Geometry: final body of the model. Coordinates: model frame, mm. A direction names the side the tool comes from. Give positions to 0.01 mm unless a question says otherwise; leave off trailing zeros. Order: outer loops, then holes, each group sorted by start corner. A loop starts at its lowest first (then second) coordinate and runs counter-clockwise, first axis right, second up. Notation, with made-up numbers: (-18, 72.5) - (3, 72.5) arc R16 ccw to (3, 82.5) - close; hole circle Ø11 at (-4.75, 46). An arc over 180 degrees is marked (long way). Put each result on its own line as item: value. Start each with the question number.
1. Ray query, line 1 along Z through (x, y) = (12.5, -39); line 2 along Z through (x, y) = (23.5, -23); line 3 along Z through (x, y) = (12.5, -76). Return the intervals inside material, ascending. Write a range as from..to.
2. Mould query, pull axis Z, two halves, no side actions, for faces 1 (the flat face through (-0.07, -31.3, 76.04)), 2 (the flat face through (2, -38, 63.522)), 3 (the flat face through (-31, -38, -7.958)). Classes: pulls with the +Z half, pulls with the -Z half, needs draft (parallel to the pull), parting line crosses it, or undercut.
3. Section B-B on z = 35. Return the cut outline in (x, y), plus the area to 3 significant figures.
4. Section D-D on z = 58.5. Return the cut outline in (x, y).
5. Section A-A on z = -17. Return the cut outline in (x, y).
6. First-contact query: P1, Ø19, axis at y = -29, z = 30.5, coming from the -X side; P2, Ø12, axis at x = 20.5, y = -21, coming from the -Z side; P3, Ø8, axis at x = 22, y = -58.5, coming from the +Z side. Flat tips, straight axial feed; report the tip coordinate or a pass-through.
7. Section C-C on z = 13.5. Return the cut outline in (x, y).
8. Set-up query: faces 4 (the flat face through (-24.5, -39.2, 88.922)), 5 (the flat face through (-26.357, -49.706, 76.044)), 6 (the flat face through (-3.93, -24.06, 76.04)), 7 (the cylindrical face through (19.688, -13.873, 31.422)). Return all of +Z, -Z, +X, -X, +Y, -Y with unobstructed straight access to the full face (end or side cutting, diameter ignored); none if empty.
from build123d import *

# Parameters (mm, degrees)
F1_DEPTH  = 76.2
F2_R      = 25.4
F3_DEPTH  = 25.4
F5_DEPTH  = 25.4
F6_R      = 10.087603
F7_DEPTH  = 25.4
F9_DEPTH  = 25.4
F10_R     = 8.870052
F11_DEPTH = 25.4
F13_DEPTH = 25.4


with BuildPart() as f1:
    # F0 (on Front) → F1 (new body)
    with BuildSketch(Plane.XZ):
        Polygon((-43.63443, -7.957917), (-43.63443, -33.357917), (32.56557, -33.357917), (32.56557, -7.957917), (7.16557, -7.957917), (7.16557, 55.542083), (30.757195, 55.542083), (30.757195, 63.522073), (-43.63443, 63.522073), (-43.63443, 55.542083), (-18.23443, 55.542083), (-18.23443, -7.957917), align=None)
    extrude(amount=F1_DEPTH)

    # F2 (on face) → F3 (join)
    with BuildSketch(Plane.YZ.offset(7.16557)):
        with Locations((-38.1, 23.792083)):
            Circle(F2_R)
    extrude(amount=F3_DEPTH)

    # F4 (on face) → F5 (join)
    with BuildSketch(Plane.XY.offset(63.522073)):
        Polygon((-0.971111, -43.576736), (0.971111, -35.34374), (-1.135201, -27.151187), (-6.807516, -20.875895), (-14.746376, -17.955455), (-23.133083, -19.058907), (-30.046344, -23.933462), (-33.902414, -31.462418), (-33.817914, -39.920983), (-29.812201, -47.371402), (-22.802937, -52.106872), (-14.395859, -53.042555), (-6.516928, -49.964097), align=None)
    extrude(amount=F5_DEPTH)

    # F6 (on face) → F7 (join)
    with BuildSketch(Plane.XY.offset(88.922073)):
        with Locations((-14.400505, -35.959587)):
            Circle(F6_R)
    extrude(amount=F7_DEPTH)

    # F8 (on face) → F9 (join)
    with BuildSketch(Plane.XZ.offset(76.2)):
        Polygon((11.728236, -26.867476), (11.728236, -27.415208), (11.811846, -27.95652), (11.977108, -28.478726), (12.220148, -28.969584), (12.535268, -29.41759), (12.915083, -29.812243), (13.35069, -30.144292), (13.831879, -30.405954), (14.347372, -30.591096), (14.885084, -30.69538), (15.432414, -30.716359), (15.976532, -30.653544), (16.504684, -30.508405), (17.004492, -30.284345), (17.464239, -29.986616), (17.87315, -29.622196), (18.22164, -29.199627), (18.501541, -28.728813), (18.706292, -28.22079), (18.831095, -27.687467), (18.873023, -27.141342), (18.831095, -26.595217), (18.706292, -26.061893), (18.501541, -25.553871), (18.22164, -25.083057), (17.87315, -24.660488), (17.464239, -24.296068), (17.004492, -23.998339), (16.504684, -23.774279), (15.976532, -23.62914), (15.432414, -23.566325), (14.885084, -23.587304), (14.347372, -23.691587), (13.831879, -23.87673), (13.35069, -24.138392), (12.915083, -24.470441), (12.535268, -24.865094), (12.220148, -25.3131), (11.977108, -25.803958), (11.811846, -26.326163), align=None)
    extrude(amount=F9_DEPTH)

    # F10 (on face) → F11 (join)
    with BuildSketch(Plane(origin=(0, 0, -33.357917), x_dir=(1, 0, 0), z_dir=(0, 0, -1))):
        with Locations((-28.388368, 46.655256)):
            Circle(F10_R)
    extrude(amount=F11_DEPTH)

    # F12 (on face) → F13 (join)
    with BuildSketch(Plane(origin=(0, 0, -33.357917), x_dir=(1, 0, 0), z_dir=(0, 0, -1))):
        with BuildLine():
            Line((9.473382, 24.02906), (9.473382, 26.472044))
            Line((9.473382, 26.472044), (9.167195, 28.895765))
            Line((9.167195, 28.895765), (8.55965, 31.261998))
            Line((8.55965, 31.261998), (7.660328, 33.533427))
            Line((7.660328, 33.533427), (6.483411, 35.67423))
            Line((6.483411, 35.67423), (5.047461, 37.650645))
            Line((5.047461, 37.650645), (3.375124, 39.431504))
            Line((3.375124, 39.431504), (1.492772, 40.988721))
            Line((1.492772, 40.988721), (-0.569908, 42.297737))
            Line((-0.569908, 42.297737), (-2.780386, 43.337909))
            Line((-2.780386, 43.337909), (-5.103801, 44.092833))
            Line((-5.103801, 44.092833), (-7.503513, 44.550602))
            Line((-7.503513, 44.550602), (-9.941677, 44.703998))
            Line((-9.941677, 44.703998), (-12.37984, 44.550602))
            Line((-12.37984, 44.550602), (-14.779552, 44.092833))
            Line((-14.779552, 44.092833), (-17.102968, 43.337909))
            Line((-17.102968, 43.337909), (-19.313446, 42.297737))
            Line((-19.313446, 42.297737), (-21.376125, 40.988721))
            Line((-21.376125, 40.988721), (-22.157084, 40.342656))
            ThreePointArc((-22.157084, 40.342656), (-22.705241, 39.844977), (-23.292994, 39.394747))
            Line((-23.292994, 39.394747), (-24.930814, 37.650645))
            Line((-24.930814, 37.650645), (-26.366764, 35.67423))
            Line((-26.366764, 35.67423), (-27.543681, 33.533427))
            Line((-27.543681, 33.533427), (-28.443003, 31.261998))
            Line((-28.443003, 31.261998), (-29.050549, 28.895765))
            Line((-29.050549, 28.895765), (-29.356736, 26.472044))
            Line((-29.356736, 26.472044), (-29.356736, 24.02906))
            Line((-29.356736, 24.02906), (-29.050549, 21.60534))
            Line((-29.050549, 21.60534), (-28.443003, 19.239107))
            Line((-28.443003, 19.239107), (-27.543681, 16.967678))
            Line((-27.543681, 16.967678), (-26.366764, 14.826875))
            Line((-26.366764, 14.826875), (-24.930814, 12.850459))
            Line((-24.930814, 12.850459), (-23.258477, 11.0696))
            Line((-23.258477, 11.0696), (-21.376125, 9.512384))
            Line((-21.376125, 9.512384), (-19.313446, 8.203367))
            Line((-19.313446, 8.203367), (-17.102968, 7.163196))
            Line((-17.102968, 7.163196), (-14.779552, 6.408272))
            Line((-14.779552, 6.408272), (-12.37984, 5.950502))
            Line((-12.37984, 5.950502), (-9.941677, 5.797106))
            Line((-9.941677, 5.797106), (-7.503513, 5.950502))
            Line((-7.503513, 5.950502), (-5.103801, 6.408272))
            Line((-5.103801, 6.408272), (-2.780386, 7.163196))
            Line((-2.780386, 7.163196), (-0.569908, 8.203367))
            Line((-0.569908, 8.203367), (1.492772, 9.512384))
            Line((1.492772, 9.512384), (3.375124, 11.0696))
            Line((3.375124, 11.0696), (5.047461, 12.850459))
            Line((5.047461, 12.850459), (6.483411, 14.826875))
            Line((6.483411, 14.826875), (7.660328, 16.967678))
            Line((7.660328, 16.967678), (8.55965, 19.239107))
            Line((8.55965, 19.239107), (9.167195, 21.60534))
            Line((9.167195, 21.60534), (9.473382, 24.02906))
        make_face()
    extrude(amount=F13_DEPTH)


solid = f1.part
Resolved:
1. line 1: -33.36..-7.96, -1.59..49.18, 55.54..63.52
1. line 2: -33.36..-7.96, 3.37..44.22, 55.54..63.52
1. line 3: -33.36..-7.96, 55.54..63.52
2. face 1: needs draft
2. face 2: pulls with the +Z half
2. face 3: undercut
3. outline: (-18.23, -76.2) - (7.17, -76.2) - (7.17, -60.89) - (32.57, -60.89) - (32.57, -15.31) - (7.17, -15.31) - (7.17, 0) - (-18.23, 0) - close
3. area: 3,090 mm^2
4. outline: (-43.63, -76.2) - (30.76, -76.2) - (30.76, 0) - (-43.63, 0) - close
5. outline: (-43.63, -76.2) - (32.57, -76.2) - (32.57, 0) - (-43.63, 0) - close
6. P1: x = -18.23
6. P2: z = -33.36
6. P3: z = 63.52
7. outline: (-18.23, -76.2) - (7.17, -76.2) - (7.17, -61.32) - (32.57, -61.32) - (32.57, -14.88) - (7.17, -14.88) - (7.17, 0) - (-18.23, 0) - close
8. face 4: +Z
8. face 5: +Z, -X, -Y
8. face 6: +Z, +X, +Y
8. face 7: +X
